```python
from build123d import *

# Parameters (mm, degrees)
BOSS_EXTRUDE1_OUTLINE_R = 16
BOSS_EXTRUDE1_DEPTH     = 60
BOSS_EXTRUDE2_START     = -60
BOSS_EXTRUDE2_DEPTH     = 60
CUT_EXTRUDE1_DEPTH      = 145.395578885
CUT_EXTRUDE2_DEPTH      = 145.395578885
SKETCH5_W               = 40
SKETCH5_H               = 37.745966692
CUT_EXTRUDE5_DEPTH      = 146.348374233
BOSS_EXTRUDE3_START     = -60
BOSS_EXTRUDE3_DEPTH     = 60
CUT_EXTRUDE6_START      = -60
SKETCH10_4_R            = 1
CUT_EXTRUDE6_DEPTH      = 60
CUT_EXTRUDE7_DEPTH      = 60
BOSS_EXTRUDE4_DEPTH     = 70
SKETCH12_W              = 7
SKETCH12_H              = 13
SKETCH12_H_2            = 7
BOSS_EXTRUDE5_DEPTH     = 62.5
SKETCH13_W              = 11
SKETCH13_H              = 2.5
CUT_EXTRUDE8_DEPTH      = 40


# Read off the part's stored shape, not the designer's step: Boss-Extrude1, Boss-Extrude3
with BuildPart() as part:
    # Boss-Extrude1 outline → Boss-Extrude1 (new body)
    with BuildSketch(Plane.XY.offset(0.755461794)):
        with Locations((-30.851105688, 17.572500308)):
            Circle(BOSS_EXTRUDE1_OUTLINE_R)
        with BuildLine():
            Line((-28.166301776, 21.908607365), (-28.260226262, 22.19606428))
            ThreePointArc((-28.260226262, 22.19606428), (-28.158199405, 22.137394146), (-28.057500467, 22.076472985))
            Line((-28.057500467, 22.076472985), (-28.166301776, 21.908607365))
        make_face(mode=Mode.SUBTRACT)
    extrude(amount=BOSS_EXTRUDE1_DEPTH)

    # Sketch2 → Boss-Extrude2 (add)
    with BuildSketch(Plane.XY.offset(60.755461794).offset(BOSS_EXTRUDE2_START)):
        with BuildLine():
            Line((-60.851105688, 17.572500308), (-46.851105688, 17.572500308))
            ThreePointArc((-46.851105688, 17.572500308), (-30.851105688, 33.572500308), (-14.851105688, 17.572500308))
            Line((-14.851105688, 17.572500308), (-14.851105688, 71.858214594))
            Line((-14.851105688, 71.858214594), (-30.851105688, 117.572500308))
            Line((-30.851105688, 117.572500308), (-60.851105688, 117.572500308))
            Line((-60.851105688, 117.572500308), (-60.851105688, 17.572500308))
        make_face()
    extrude(amount=BOSS_EXTRUDE2_DEPTH)

    # Sketch3 → Cut-Extrude1 (cut, through all)
    with BuildSketch(Plane(origin=(0, 117.572500308, 0), x_dir=(1, 0, 0), z_dir=(0, 1, 0))):
        with BuildLine():
            Line((-60.851105688, -29.505461794), (-60.851105688, -32.005461794))
            Line((-60.851105688, -32.005461794), (-53.678502861, -32.005461794))
            ThreePointArc((-53.678502861, -32.005461794), (-52.758859998, -31.502501818), (-51.839217136, -32.005461794))
            Line((-51.839217136, -32.005461794), (-49.851105688, -32.005461794))
            Line((-49.851105688, -32.005461794), (-49.851105688, -29.505461794))
            Line((-49.851105688, -29.505461794), (-51.839217136, -29.505461794))
            ThreePointArc((-51.839217136, -29.505461794), (-52.758859998, -30.00842177), (-53.678502861, -29.505461794))
            Line((-53.678502861, -29.505461794), (-60.851105688, -29.505461794))
        make_face()
    extrude(amount=-CUT_EXTRUDE1_DEPTH, mode=Mode.SUBTRACT)

    # Sketch4 → Cut-Extrude2 (cut, through all)
    with BuildSketch(Plane(origin=(0, 117.572500308, 0), x_dir=(1, 0, 0), z_dir=(0, 1, 0))):
        Polygon((-60.851105688, -27.255461794), (-44.851105688, -0.755461794), (-60.851105688, -0.755461794), align=None)
        Polygon((-60.851105688, -34.255461794), (-44.851105688, -60.755461794), (-60.851105688, -60.755461794), align=None)
    extrude(amount=-CUT_EXTRUDE2_DEPTH, mode=Mode.SUBTRACT)

    # Sketch5 → Cut-Extrude5 (cut, through all)
    with BuildSketch(Plane(origin=(0, 0, 0.755461794), x_dir=(-1, 0, 0), z_dir=(0, 0, -1))):
        with Locations((64.851105688, 28.699516962)):
            Rectangle(SKETCH5_W, SKETCH5_H)
    extrude(amount=-CUT_EXTRUDE5_DEPTH, mode=Mode.SUBTRACT)

    # Boss-Extrude3 outline → Boss-Extrude3 (add)
    with BuildSketch(Plane.XY.offset(60.755461794).offset(BOSS_EXTRUDE3_START)):
        with BuildLine():
            ThreePointArc((-14.851105688, 17.572500308), (-24.419989547, 2.92187762), (-41.681198835, 5.795018301))
            ThreePointArc((-41.681198835, 5.795018301), (-2.90297286, 3.119259484), (-14.851105688, 40.107806589))
            Line((-14.851105688, 40.107806589), (-14.851105688, 17.572500308))
        make_face()
    extrude(amount=BOSS_EXTRUDE3_DEPTH)

    # Sketch10<4> → Cut-Extrude6 (cut)
    with BuildSketch(Plane.XY.offset(60.755461794).offset(CUT_EXTRUDE6_START)):
        with BuildLine():
            ThreePointArc((-44.851105688, 9.826533616), (-43.428731074, 7.682943208), (-41.681198835, 5.795018301))
            ThreePointArc((-41.681198835, 5.795018301), (-44.044774342, 11.474193332), (-44.851105688, 17.572500308))
            Line((-44.851105688, 17.572500308), (-44.851105688, 9.826533616))
        make_face()
        with BuildLine():
            ThreePointArc((-40.851105688, 17.572500308), (-39.851105688, 16.572500308), (-38.851105688, 17.572500308))
            Line((-38.851105688, 17.572500308), (-40.851105688, 17.572500308))
        make_face()
        with BuildLine():
            Line((-40.851105688, 17.572500308), (-38.851105688, 17.572500308))
            ThreePointArc((-38.851105688, 17.572500308), (-39.851105688, 18.572500308), (-40.851105688, 17.572500308))
        make_face()
        with BuildLine():
            ThreePointArc((-20.387105202, -0.891500177), (-20.679998421, -0.184393396), (-21.387105202, 0.108499823))
            Line((-21.387105202, 0.108499823), (-21.387105202, -1.891500177))
            ThreePointArc((-21.387105202, -1.891500177), (-20.679998421, -1.598606959), (-20.387105202, -0.891500177))
        make_face()
        with BuildLine():
            Line((-21.387105202, -1.891500177), (-21.387105202, 0.108499823))
            ThreePointArc((-21.387105202, 0.108499823), (-22.387105202, -0.891500177), (-21.387105202, -1.891500177))
        make_face()
        with BuildLine():
            ThreePointArc((-2.923104717, 18.572500308), (-3.630211498, 18.27960709), (-3.923104717, 17.572500308))
            Line((-3.923104717, 17.572500308), (-2.923104717, 17.572500308))
            Line((-2.923104717, 17.572500308), (-2.923104717, 18.572500308))
        make_face()
        with BuildLine():
            Line((-2.923104717, 17.572500308), (-3.923104717, 17.572500308))
            ThreePointArc((-3.923104717, 17.572500308), (-2.923104717, 16.572500308), (-1.923104717, 17.572500308))
            ThreePointArc((-1.923104717, 17.572500308), (-2.215997935, 18.27960709), (-2.923104717, 18.572500308))
            Line((-2.923104717, 18.572500308), (-2.923104717, 17.572500308))
        make_face()
        with Locations((-21.387105202, 36.036500794)):
            Circle(SKETCH10_4_R)
    extrude(amount=CUT_EXTRUDE6_DEPTH, mode=Mode.SUBTRACT)

    # Sketch10<5> → Cut-Extrude7 (cut)
    # profile 1 of 6: a face of its own
    with BuildSketch(Plane.XY.offset(60.755461794)):
        with BuildLine():
            ThreePointArc((-14.851105688, 17.572500308), (-16.578334273, 10.341456392), (-21.387105202, 4.671620695))
            Line((-21.387105202, 4.671620695), (-21.387105202, 2.572500308))
            ThreePointArc((-21.387105202, 2.572500308), (-10.780503485, 6.965898591), (-6.387105202, 17.572500308))
            Line((-6.387105202, 17.572500308), (-14.851105688, 17.572500308))
        make_face()
    # profile 2 of 6: a face of its own
    with BuildSketch(Plane.XY.offset(60.755461794)):
        with BuildLine():
            Line((-14.851105688, 31.073637681), (-14.851105688, 17.572500308))
            Line((-14.851105688, 17.572500308), (-6.387105202, 17.572500308))
            ThreePointArc((-6.387105202, 17.572500308), (-8.678053454, 25.539934252), (-14.851105688, 31.073637681))
        make_face()
    # profile 3 of 6: a face of its own
    with BuildSketch(Plane.XY.offset(60.755461794)):
        with BuildLine():
            Line((-30.851105688, 17.572500308), (-21.387105202, 17.572500308))
            Line((-21.387105202, 17.572500308), (-14.851105688, 17.572500308))
            Line((-14.851105688, 17.572500308), (-14.851105688, 31.073637681))
            ThreePointArc((-14.851105688, 31.073637681), (-29.354539146, 30.281552057), (-36.387105202, 17.572500308))
            Line((-36.387105202, 17.572500308), (-30.851105688, 17.572500308))
        make_face()
        with BuildLine():
            Line((-28.166301776, 21.908607365), (-28.260226262, 22.19606428))
            ThreePointArc((-28.260226262, 22.19606428), (-28.158199405, 22.137394146), (-28.057500467, 22.076472985))
            Line((-28.057500467, 22.076472985), (-28.166301776, 21.908607365))
        make_face(mode=Mode.SUBTRACT)
    # profile 4 of 6: a face of its own
    with BuildSketch(Plane.XY.offset(60.755461794)):
        with BuildLine():
            Line((-14.851105688, 17.572500308), (-21.387105202, 17.572500308))
            Line((-21.387105202, 17.572500308), (-21.387105202, 4.671620695))
            ThreePointArc((-21.387105202, 4.671620695), (-16.578334273, 10.341456392), (-14.851105688, 17.572500308))
        make_face()
    # profile 5 of 6: a face of its own
    with BuildSketch(Plane.XY.offset(60.755461794)):
        with BuildLine():
            Line((-21.387105202, 4.671620695), (-21.387105202, 17.572500308))
            Line((-21.387105202, 17.572500308), (-30.851105688, 17.572500308))
            Line((-30.851105688, 17.572500308), (-36.387105202, 17.572500308))
            ThreePointArc((-36.387105202, 17.572500308), (-33.036423327, 8.122982478), (-24.481320238, 2.895108397))
            ThreePointArc((-24.481320238, 2.895108397), (-22.884538469, 3.696845126), (-21.387105202, 4.671620695))
        make_face()
    # profile 6 of 6: a face of its own
    with BuildSketch(Plane.XY.offset(60.755461794)):
        with BuildLine():
            Line((-21.387105202, 2.572500308), (-21.387105202, 4.671620695))
            ThreePointArc((-21.387105202, 4.671620695), (-22.884538469, 3.696845126), (-24.481320238, 2.895108397))
            ThreePointArc((-24.481320238, 2.895108397), (-22.942598907, 2.653370329), (-21.387105202, 2.572500308))
        make_face()
    extrude(amount=-CUT_EXTRUDE7_DEPTH, mode=Mode.SUBTRACT)

    # Sketch11 → Boss-Extrude4 (add)
    with BuildSketch(Plane(origin=(0, 117.572500308, 0), x_dir=(1, 0, 0), z_dir=(0, 1, 0))):
        Polygon((-44.851105688, -0.755461794), (-60.851105688, -0.755461794), (-60.851105688, -27.255461794), align=None)
        Polygon((-60.851105688, -34.255461794), (-60.851105688, -60.755461794), (-44.851105688, -60.755461794), align=None)
    extrude(amount=-BOSS_EXTRUDE4_DEPTH)

    # Sketch12 → Boss-Extrude5 (add)
    with BuildSketch(Plane(origin=(0, 117.572500308, 0), x_dir=(1, 0, 0), z_dir=(0, 1, 0))):
        with Locations((-64.351105688, -7.255461794)):
            Rectangle(SKETCH12_W, SKETCH12_H)
        with Locations((-64.351105688, -57.255461794)):
            Rectangle(SKETCH12_W, SKETCH12_H_2)
    extrude(amount=-BOSS_EXTRUDE5_DEPTH)

    # Sketch13 → Cut-Extrude8 (cut)
    with BuildSketch(Plane.XZ.offset(-47.572500308)):
        with Locations((-55.351105688, 30.755461794)):
            Rectangle(SKETCH13_W, SKETCH13_H)
    extrude(amount=-CUT_EXTRUDE8_DEPTH, mode=Mode.SUBTRACT)


solid = part.part
```
Here's how the part is built. I have some questions about the finished solid (model axes, mm). A direction names the side the tool comes from. Give positions to 0.01 mm unless a question says otherwise; leave off trailing zeros. Write each loop counter-clockwise with the first axis right and the second up, starting at its lowest first coordinate (ties: lowest second). Pieces come first, ordered by that corner, then holes. Notation, with made-up numbers: (-4.75, -31) -> (34.25, -31) arc R19 ccw to (34.25, 3) -> close; hole circle Ø1 at (38, -27.75). An arc over 180 degrees is marked (long way). Write each question's results on one line, items separated by ' | '.
Item 1: Suppose I cut it at D-D on y = 23.5. Write out the boundary of the cut face in (x, z).
Output:
outline: (-44.85, 0.76) -> (-35.17, 0.76) -> (-35.17, 60.76) -> (-44.85, 60.76) -> close; (-7.61, 0.76) -> (1.32, 0.76) -> (1.32, 60.76) -> (-7.61, 60.76) -> close
Item 2: Suppose I cut it at A-A on x = -58. Write out the boundary of the cut face in (y, z), plus the area to 4 significant figures.
Output:
outline: (47.57, 0.76) -> (117.57, 0.76) -> (117.57, 29.51) -> (47.57, 29.51) -> close; (47.57, 32.01) -> (117.57, 32.01) -> (117.57, 60.76) -> (47.57, 60.76) -> close | area: 4,025 mm^2
Item 3: Suppose I cut it at C-C on y = 62. Write out the boundary of the cut face in (x, z), plus the area to 3 significant figures.
Output:
outline: (-67.85, 0.76) -> (-14.85, 0.76) -> (-14.85, 60.76) -> (-67.85, 60.76) -> (-67.85, 53.76) -> (-60.85, 53.76) -> (-60.85, 32.01) -> (-49.85, 32.01) -> (-49.85, 29.51) -> (-60.85, 29.51) -> (-60.85, 13.76) -> (-67.85, 13.76) -> close | area: 2,870 mm^2
Item 4: We'd pull the mould along Z, two halves only. Please class faces 1 (the face through (-41, 70, 60.755)), 2 (the face through (-45, 117.573, 30)), 3 (the face through (-64, 87, 13.755)), 4 (the face through (-60.851, 83, 43)): pulls with the +Z half, pulls with the -Z half, needs draft (parallel to the pull), parting line crosses it, or undercut.
Output:
face 1: pulls with the +Z half | face 2: needs draft | face 3: undercut | face 4: undercut
Item 5: Suppose I cut it at B-B on z = 52. Write out the boundary of the cut face in (x, y), plus the area to 3 significant figures.
Output:
outline: (-60.85, 47.57) -> (-44.85, 47.57) -> (-44.85, 17.57) arc R23.46 ccw (long way) to (-14.85, 40.11) -> (-14.85, 71.86) -> (-30.85, 117.57) -> (-60.85, 117.57) -> close; hole circle Ø2 at (-39.85, 17.57); hole circle Ø30 at (-21.39, 17.57); hole circle Ø2 at (-21.39, -0.89); hole circle Ø2 at (-21.39, 36.04); hole circle Ø2 at (-2.92, 17.57) | area: 4,180 mm^2
Item 6: For pin 1 Ø3 at (y, z) = (93.5, 31) entering from -X; pin 2 Ø8 at (y, z) = (21, 53) entering from -X; pin 3 Ø4 at (y, z) = (42.5, 43) entering from +X, each with a flat end and sliding along its axis, tell me the tip position at first contact or that it passes through.
Output:
pin 1: stops at x = -60.85 | pin 2: stops at x = -44.85 | pin 3: stops at x = -14.85
Item 7: If I drill on L1, parallel to Y at x = -52, z = 36; L2, parallel to X at y = 14.5, z = 5; L3, parallel to X at y = 36.5, z = 36, over which ranges is the centre line in solid material (lowest first)?
Output:
L1: y = 47.57 to 117.57 | L2: x = -44.65 to -36.07, -6.71 to 1.87 | L3: x = -44.85 to -22.27, -20.5 to -7.52
Item 8: On a 3-axis mill with a long thin cutter (end or side, diameter ignored), from which of +Z, -Z, +X, -X, +Y, -Y can I reach the whole of each face in a straight line? I mean faces 5 (the face through (-64, 87, 53.755)), 6 (the face through (-14.851, 56, 30)), 7 (the face through (-49.851, 83, 31)), 8 (the face through (-44.851, 32, 30)), 9 (the face through (-67.851, 87, 57)). Say none if no direction works.
Output:
face 5: -X, +Y, -Y | face 6: +Z, -Z, +X, +Y | face 7: +Y, -Y | face 8: +Z, -Z, -X, -Y | face 9: +Z, -Z, -X, +Y, -Y
